Autodesk Fusion 360 part; units mm, degrees
sketch "Sketch1" plane through (0, 0, 0) normal (0, 0, 1) x (1, 0, 0)
  line L0 (0, 0) -> (80, 0)
  line L1 (80, 0) -> (80, 110)
  line L2 (80, 110) -> (0, 110)
  line L3 (0, 110) -> (0, 0)
  dimension "d1" = 80
  dimension "d2" = 110
extrude "Extrude1" add sketch "Sketch1" along normal blind 5
fillet "Fillet1" radius 5 4 edges at (80, 0, 2.5) (0, 0, 2.5) (80, 110, 2.5) (0, 110, 2.5)
sketch "Sketch2" plane through (0, 0, 5) normal (0, 0, 1) x (-1, 0, 0)
  arc A0 (-5, -110) -> (0, -105) centre (-5, -105) ccw
  line L0 (0, -105) -> (0, -5)
  arc A1 (0, -5) -> (-5, 0) centre (-5, -5) ccw
  line L1 (-5, 0) -> (-75, 0)
  arc A2 (-75, 0) -> (-80, -5) centre (-75, -5) ccw
  line L2 (-80, -5) -> (-80, -105)
  arc A3 (-80, -105) -> (-75, -110) centre (-75, -105) ccw
  line L3 (-75, -110) -> (-5, -110)
  line L4 (-5, -30) -> (-8, -30)
  line L5 (-8, -30) -> (-8, -20)
  line L6 (-8, -20) -> (-5, -20)
  line L7 (-5, -20) -> (-5, -30)
  line L8 (-5, -90) -> (-8, -90)
  line L9 (-8, -90) -> (-8, -80)
  line L10 (-8, -80) -> (-5, -80)
  line L11 (-5, -80) -> (-5, -90)
  line L12 (0, 0) -> (-40, 0)
  line L13 (-40, 0) -> (-40, -110)
  line L14 (-75, -90) -> (-72, -90)
  line L15 (-72, -90) -> (-72, -80)
  line L16 (-75, -80) -> (-75, -90)
  line L17 (-72, -80) -> (-75, -80)
  line L18 (-75, -30) -> (-72, -30)
  line L19 (-72, -20) -> (-75, -20)
  line L20 (-75, -20) -> (-75, -30)
  line L21 (-72, -30) -> (-72, -20)
  dimension "d7" = 3
  dimension "d8" = 10
  dimension "d9" = 3
  dimension "d10" = 10
  dimension "d11" = 5
  dimension "d12" = 5
  dimension "d13" = 20
  dimension "d14" = 20
  dimension "d15" = 40
extrude "Extrude2" add sketch "Sketch2" along normal blind 7.5 contours L4 L5 L6 L7 | L8 L9 L10 L11 | L14 L15 L16 L17 | L18 L19 L20 L21
sketch "Sketch3" plane through (0, 20, 0) normal (0, -1, 0) x (1, 0, 0)
  line L0 (5, 5) -> (8, 5)
  line L1 (8, 5) -> (8, 12.5)
  line L2 (8, 12.5) -> (5, 12.5)
  line L3 (5, 12.5) -> (5, 5)
  line L4 (5, 12.5) -> (2, 12.5)
  line L5 (8, 12.5) -> (8, 17.5)
  line L6 (8, 17.5) -> (2, 12.5)
  line L7 (72, 12.5) -> (72, 17.5)
  line L8 (75, 12.5) -> (78, 12.5)
  line L9 (72, 17.5) -> (78, 12.5)
  line L10 (72, 12.5) -> (75, 12.5)
  dimension "d18" = 5
  dimension "d48" = 3
  dimension "d54" = 5
  dimension "d55" = 3
extrude "Extrude3" add sketch "Sketch3" against normal blind 10 contours L2 L4 L5 L6 | L7 L8 L9 L10
sketch "Sketch4" plane through (0, 90, 0) normal (0, 1, 0) x (-1, 0, 0)
  line L0 (-75, 5) -> (-72, 5)
  line L1 (-72, 5) -> (-72, 12.5)
  line L2 (-72, 12.5) -> (-75, 12.5)
  line L3 (-75, 12.5) -> (-75, 5)
  line L4 (-78, 12.5) -> (-72, 17.5)
  line L5 (-72, 17.5) -> (-72, 12.5)
  line L6 (-78, 12.5) -> (-75, 12.5)
  line L7 (-8, 12.5) -> (-5, 12.5)
  line L8 (-5, 12.5) -> (-2, 12.5)
  line L9 (-8, 12.5) -> (-8, 17.5)
  line L10 (-8, 17.5) -> (-2, 12.5)
  dimension "d42" = 5
  dimension "d43" = 3
  dimension "d46" = 3
  dimension "d47" = 3
  dimension "d52" = 5
extrude "Extrude4" add sketch "Sketch4" against normal blind 10 contours L2 L4 L5 L6 | L7 L8 L9 L10
sketch "Sketch9" plane through (0, 90, 0) normal (0, 1, 0) x (-1, 0, 0)
  line L0 (-75, 5) -> (-72, 5)
  line L1 (-72, 5) -> (-72, 17.5)
  line L2 (-72, 17.5) -> (-78, 12.5)
  line L3 (-78, 12.5) -> (-75, 12.5)
  line L4 (-75, 12.5) -> (-75, 5)
  line L5 (-72, 17.5) -> (-76.5, 17.5)
  line L6 (-76.5, 17.5) -> (-78, 12.5)
  line L7 (-72, 17.5) -> (-73, 17.5)
  line L8 (-73, 17.5) -> (-73, 5)
  line L9 (-73, 5) -> (-72, 5)
  line L10 (-72, 5) -> (-72, 17.5)
  line L11 (-73, 16.6667) -> (-76.75, 16.6667)
  dimension "d56" = 4.5
  dimension "d57" = 1
sketch "Sketch10" plane through (0, 90, 0) normal (0, 1, 0) x (-1, 0, 0)
  line L0 (-8, 5) -> (-5, 5)
  line L1 (-5, 5) -> (-5, 12.5)
  line L2 (-5, 12.5) -> (-2, 12.5)
  line L3 (-2, 12.5) -> (-8, 17.5)
  line L4 (-8, 17.5) -> (-8, 5)
  line L5 (-8, 17.5) -> (-3.5, 17.5)
  line L6 (-3.5, 17.5) -> (-2, 12.5)
  line L7 (-8, 17.5) -> (-7, 17.5)
  line L8 (-7, 17.5) -> (-7, 5)
  line L9 (-7, 5) -> (-8, 5)
  line L10 (-8, 5) -> (-8, 17.5)
  line L11 (-7, 16.6667) -> (-3.25, 16.6667)
  dimension "d58" = 4.5
  dimension "d59" = 1
extrude "Extrude8" cut sketch "Sketch10" sketch "Sketch9" against normal blind 70 contours L0 L3 L4 L8 L9 L10 | L3 L5 L7 L8 of sketch 2 contours L0 L1 L2 L8 L9 L10 | L2 L5 L7 L8
extrude "Extrude9" add sketch "Sketch10" sketch "Sketch9" against normal blind 70 contours L3 L6 L11 of sketch 2 contours L2 L6 L11
sketch "Sketch11" plane through (0, 0, 0) normal (-1, 0, 0) x (0, -1, 0)
  line L0 (-105, 5) -> (-105, 0)
  line L1 (-105, 0) -> (-5, 0)
  line L2 (-5, 0) -> (-5, 5)
  line L3 (-5, 5) -> (-105, 5)
  line L4 (-110, 5) -> (-80, 5)
  line L5 (-80, 5) -> (-30, 5)
  line L6 (-30, 5) -> (-30, 26)
  line L7 (-30, 26) -> (-80, 26)
  line L8 (-80, 26) -> (-80, 5)
  dimension "d64" = 50
extrude "Extrude10" cut sketch "Sketch11" against normal blind 100 contours L3 L5 L6 L7 L8
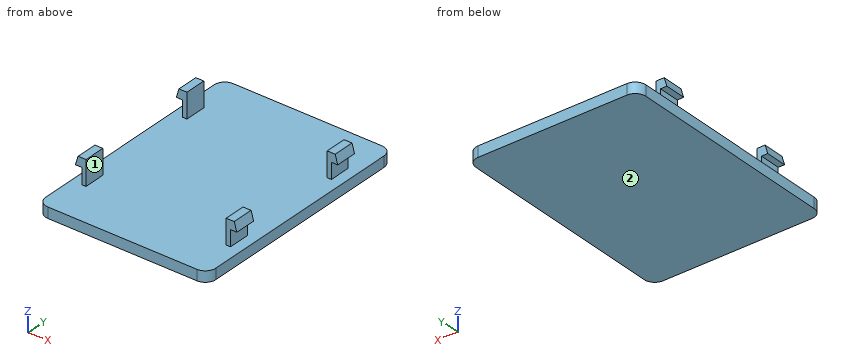
Work out the finished part from the listing and answer in its coordinate system (mm). Face numbers are marked on the shaded views. Give positions to 0.01 mm unless a question says otherwise; leave off trailing zeros. Loops run counter-clockwise (first coordinate to the right, second up) from the corner with the lowest first, then second, coordinate; pieces in that order, holes last. Notation, with made-up numbers: (88, -29.75) -> (132, -29.75) arc R8 cw to (132, -16.75) -> close; hole circle Ø8 at (65.25, 79.25). An arc over 180 degrees is marked (long way). Put each result on its own line as item: value. Start each with the question number.
Item 1: The part is cut by section B-B (y = 88.5). Give the vertices of the cut face in (x, z).
Item 2: Find the intervals of material crossed by L1, parallel to Y at x = 74.5, z = 12.75; L2, parallel to X at y = 20.5, z = 9.5; L3, parallel to Z at x = 38.5, y = 37, in increasing order. Write a range as [from, to].
Item 3: Each of these flat-tipped pins is pushed along its axis until it touches: P1, Ø10, axis at y = 88.5, z = 12.5, coming from the -X side; P2, Ø5.5, axis at x = 75.5, z = 11.5, coming from the -Y side; P3, Ø2, axis at y = 22.5, z = 7, coming from the -X side; P4, Ø2, axis at x = 16.5, y = 29.5, coming from the -Z side. Where does it stop, or does it pass through?
Item 4: The part is cut by section D-D (x = 60.5). Give the vertices of the cut face in (y, z), then the cut area to 3 significant figures.
Item 5: The part is cut by section C-C (z = 15). Give the vertices of the cut face in (x, y), then the cut area to 3 significant figures.
Item 6: The mould has two halves that part along X. Classify the marked faces 1 and 2: released by +X, released by -X, zero draft, split by the parting line, or undercut.
Item 7: The part is cut by section A-A (z = 7). Give the vertices of the cut face in (x, y).
Answers below:
1. outline: (0, 0) -> (80, 0) -> (80, 5) -> (75, 5) -> (75, 12.5) -> (78, 12.5) -> (76.75, 16.67) -> (73, 16.67) -> (73, 5) -> (7, 5) -> (7, 16.67) -> (3.25, 16.67) -> (2, 12.5) -> (5, 12.5) -> (5, 5) -> (0, 5) -> close
2. L1: [20, 30], [80, 90]
2. L2: [5, 7], [73, 75]
2. L3: [0, 5]
3. P1: x = 2
3. P2: y = 20
3. P3: x = 5
3. P4: z = 0
4. outline: (0, 0) -> (110, 0) -> (110, 5) -> (0, 5) -> close
4. area: 550 mm2
5. outline: (2.75, 20) -> (7, 20) -> (7, 30) -> (2.75, 30) -> close; (2.75, 80) -> (7, 80) -> (7, 90) -> (2.75, 90) -> close; (73, 20) -> (77.25, 20) -> (77.25, 30) -> (73, 30) -> close; (73, 80) -> (77.25, 80) -> (77.25, 90) -> (73, 90) -> close
5. area: 170 mm2
6. face 1: undercut
6. face 2: zero draft
7. outline: (5, 20) -> (7, 20) -> (7, 30) -> (5, 30) -> close; (5, 80) -> (7, 80) -> (7, 90) -> (5, 90) -> close; (73, 20) -> (75, 20) -> (75, 30) -> (73, 30) -> close; (73, 80) -> (75, 80) -> (75, 90) -> (73, 90) -> close
